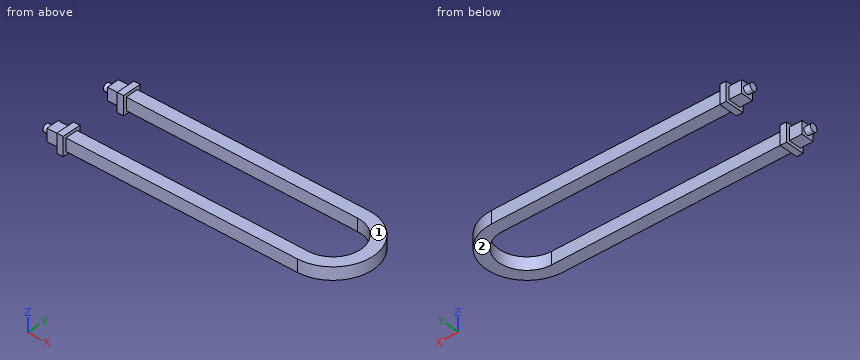
```python
from build123d import *

# Parameters (mm, degrees)
BOSS_EXTRUDE1_DEPTH   = 10
SKETCH2_R             = 3
BOSS_EXTRUDE2_DEPTH   = 15
SKETCH3_R             = 3
BOSS_EXTRUDE3_DEPTH   = 15
SKETCH5_W             = 15
SKETCH5_H             = 15
BOSS_EXTRUDE4_DEPTH   = 5
BOSS_EXTRUDE4_2_DEPTH = 5
SKETCH7_W             = 10
SKETCH7_H             = 10
BOSS_EXTRUDE5_DEPTH   = 10


with BuildPart() as part:
    # Sketch1 → Boss-Extrude1 (new body)
    with BuildSketch(Plane.XY):
        with BuildLine():
            Line((0, 0), (188.467924539, 0))
            ThreePointArc((188.467924539, 0), (220.672766762, -32.204842223), (188.467924539, -64.409684446))
            Line((188.467924539, -64.409684446), (0, -64.409684446))
            Line((0, -64.409684446), (0, -54.409684446))
            Line((0, -54.409684446), (188.467924539, -54.409684446))
            ThreePointArc((188.467924539, -54.409684446), (210.672766762, -32.204842223), (188.467924539, -10))
            Line((188.467924539, -10), (0, -10))
            Line((0, -10), (0, 0))
        make_face()
    extrude(amount=BOSS_EXTRUDE1_DEPTH)

    # Sketch2 → Boss-Extrude2 (add)
    with BuildSketch(Plane.ZY):
        with Locations(Location((5, -4.906979909, 0), (0, 0, 180))):
            Circle(SKETCH2_R)
    extrude(amount=BOSS_EXTRUDE2_DEPTH)



with BuildPart() as body_2:
    # Sketch3 → Boss-Extrude3 (new body)
    with BuildSketch(Plane.ZY):
        with Locations((5, -59.409684446)):
            Circle(SKETCH3_R)
    extrude(amount=BOSS_EXTRUDE3_DEPTH)


with BuildPart() as body_3:
    # Sketch5 → Boss-Extrude4 (new body)
    with BuildSketch(Plane(origin=(0, 0, 0), x_dir=(0, 0, -1), z_dir=(1, 0, 0))):
        with Locations((-5, -59.409684446)):
            Rectangle(SKETCH5_W, SKETCH5_H)
    extrude(amount=BOSS_EXTRUDE4_DEPTH)


with BuildPart() as body_4:
    # Sketch5 → Boss-Extrude4 2 (new body)
    with BuildSketch(Plane(origin=(0, 0, 0), x_dir=(0, 0, -1), z_dir=(1, 0, 0))):
        with Locations((-5, -5)):
            Rectangle(SKETCH5_W, SKETCH5_H)
    extrude(amount=BOSS_EXTRUDE4_2_DEPTH)


with BuildPart() as part_1:
    add(part.part)

    add(body_2.part)  # Boss-Extrude5 merges body 2

    add(body_3.part)  # Boss-Extrude5 merges body 3

    add(body_4.part)  # Boss-Extrude5 merges body 4
    # Sketch7 → Boss-Extrude5 (add)
    with BuildSketch(Plane.ZY):
        with Locations((5, -59.502704537)):
            Rectangle(SKETCH7_W, SKETCH7_H)
        with Locations((5, -4.906979909)):
            Rectangle(SKETCH7_W, SKETCH7_H)
    extrude(amount=BOSS_EXTRUDE5_DEPTH)


solid = part_1.part
```
Could you check a few things on this model? Use its own coordinates, in mm. Face numbers are marked on the shaded views. A direction names the side the tool comes from. Coordinates: 2 decimals unless noted, no trailing zeros. Write each loop counter-clockwise with the first axis right and the second up, starting at its lowest first coordinate (ties: lowest second). Pieces come first, ordered by that corner, then holes. Notation, with made-up numbers: (11.25, 56.5) -> (36.25, 56.5) arc R12 cw to (36.25, 79.5) -> close; hole circle Ø11 at (41.5, -2.75). An arc over 180 degrees is marked (long way). Return JSON: item names as keys, results as strings.
(1) Imagine slicing it at A-A, the plane x = 149. Please give me the cut outline in (y, z).
Numbers:
{"outline": "(-64.41, 0) -> (-54.41, 0) -> (-54.41, 10) -> (-64.41, 10) -> close; (-10, 0) -> (0, 0) -> (0, 10) -> (-10, 10) -> close"}
(2) Which directions (+Z, -Z, +X, -X, +Y, -Y) give clear straight access to the entire face, cutting with the end or side of a thin tool? Please do the marked faces 1 and 2.
Numbers:
{"face 1": "+Z, +X, +Y, -Y", "face 2": "-Z, +X, +Y, -Y"}
(3) Imagine slicing it at C-C, the plane x = 201.5. Please give me the cut outline in (y, z).
Numbers:
{"outline": "(-61.66, 0) -> (-50.18, 0) -> (-50.18, 10) -> (-61.66, 10) -> close; (-14.23, 0) -> (-2.75, 0) -> (-2.75, 10) -> (-14.23, 10) -> close"}
(4) I'm going to push flat-ended pins straight in: pin 1 (1.5 mm diameter, centred on x = 182.5, z = 2, fed in from -Y); pin 2 (7.5 mm diameter, centred on y = -3, z = 6, fed in from +X); pin 3 (3 mm diameter, centred on x = 122.5, z = 7, fed in from +Y). Where does each tip first touch, or does it pass through?
Numbers:
{"pin 1": "stops at y = -64.41", "pin 2": "stops at x = 208.2", "pin 3": "stops at y = 0"}
(5) I need wall thicknesses on L1, parallel to Y at x = 99, z = 1.25; L2, parallel to Z at x = 76.5, y = -55; L3, parallel to X at y = -64, z = 10.25. Which ranges of each line are inside material? Lowest first, please.
Numbers:
{"L1": "y = -64.41 to -54.41, -10 to 0", "L2": "z = 0 to 10", "L3": "x = 0 to 5"}
(6) Imagine slicing it at D-D, the plane y = -27. Please give me the cut outline in (x, z), then the cut area to 3 significant figures.
Numbers:
{"outline": "(210.05, 0) -> (220.25, 0) -> (220.25, 10) -> (210.05, 10) -> close", "area": "102 mm2"}
